CAD build for the part. Positions are in the model's coordinates, mm. Face numbers are marked on the shaded views. A direction names the side the tool comes from. Coordinates: 2 decimals unless noted, no trailing zeros. Loops run counter-clockwise (first coordinate to the right, second up) from the corner with the lowest first, then second, coordinate; pieces in that order, holes last. Notation, with made-up numbers: (-29.75, 51) -> (-25.75, 51) arc R31 cw to (-25.75, 86) -> close; hole circle Ø10 at (84, 88). An arc over 180 degrees is marked (long way). Write each question's results on one line, items separated by ' | '.
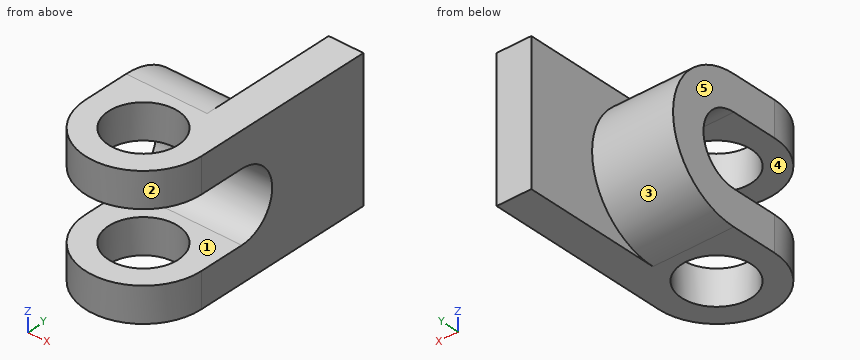
```python
from build123d import *

# Parameters (mm, degrees)
SKETCH1_R           = 15
BOSS_EXTRUDE1_DEPTH = 60
BOSS_EXTRUDE2_DEPTH = 35
CUT_EXTRUDE9_DEPTH  = 68


with BuildPart() as part:
    # Sketch1 → Boss-Extrude1 (new body)
    with BuildSketch(Plane.XY):
        with BuildLine():
            Line((25, 0), (25, 80))
            Line((25, 80), (10, 80))
            Line((10, 80), (10, 20))
            Line((10, 20), (-25, 20))
            Line((-25, 20), (-25, 0))
            ThreePointArc((-25, 0), (0, -25), (25, 0))
        make_face()
        Circle(SKETCH1_R, mode=Mode.SUBTRACT)
    extrude(amount=BOSS_EXTRUDE1_DEPTH)

    # Sketch2 → Boss-Extrude2 (add)
    with BuildSketch(Plane.ZY.offset(25)):
        with BuildLine():
            Line((15, 20), (0, 20))
            ThreePointArc((0, 20), (30, 50), (60, 20))
            Line((60, 20), (45, 20))
            ThreePointArc((45, 20), (30, 35), (15, 20))
        make_face()
    extrude(amount=-BOSS_EXTRUDE2_DEPTH)

    # Sketch4 → Cut-Extrude9 (cut)
    with BuildSketch(Plane.ZY.offset(25)):
        with BuildLine():
            Line((15, 20), (15, -31.386315339))
            Line((15, -31.386315339), (45, -31.386315339))
            Line((45, -31.386315339), (45, 20))
            ThreePointArc((45, 20), (30, 35), (15, 20))
        make_face()
    extrude(amount=-CUT_EXTRUDE9_DEPTH, mode=Mode.SUBTRACT)


solid = part.part
```
Q1. Pull direction Z, two halves, no side cores. Call the marked faces 1, 2 and 3: +Z half, -Z half, draft (parallel to the pull), parting line (faces both ways), or undercut.
Results are:
face 1: undercut | face 2: draft | face 3: parting line
Q2. Cut at C-C on z = 9.5. Write the cut outline in (x, y), and give its area (3 significant figures).
Results are:
outline: (-25, 0) arc R25 ccw to (25, 0) -> (25, 80) -> (10, 80) -> (10, 41.9) -> (-25, 41.9) -> close; hole circle Ø30 at (0, 0) | area: 2,940 mm^2
Q3. Wall check: L1, parallel to Z at x = 10, y = -14; L2, parallel to X at y = 0, z = 55; L3, parallel to Y at x = 0, z = 52.5. Give the ranges that are in metal, low to high. Write a range as from..to.
Results are:
L1: 0..15, 45..60 | L2: -25..-15, 15..25 | L3: -25..-15, 15..39.84
Q4. Cut at A-A on x = 0. Write the cut outline in (y, z).
Results are:
outline: (-25, 0) -> (-15, 0) -> (-15, 15) -> (-25, 15) -> close; (-25, 45) -> (-15, 45) -> (-15, 60) -> (-25, 60) -> close; (15, 0) -> (20, 0) arc R30 ccw to (20, 60) -> (15, 60) -> (15, 45) -> (20, 45) arc R15 cw to (20, 15) -> (15, 15) -> close
Q5. Drop a flat-ended pin along its axis: pin 1 (12 mm diameter, centred on x = -18, z = 46.5, fed in from +Y). Give the stop position or say it passes through.
Results are:
pin 1: y = 48.1
Q6. Cut at B-B on y = -11. Write the cut outline in (x, z), and give its area (3 significant figures).
Results are:
outline: (-22.45, 0) -> (-10.2, 0) -> (-10.2, 15) -> (-22.45, 15) -> close; (-22.45, 45) -> (-10.2, 45) -> (-10.2, 60) -> (-22.45, 60) -> close; (10.2, 0) -> (22.45, 0) -> (22.45, 15) -> (10.2, 15) -> close; (10.2, 45) -> (22.45, 45) -> (22.45, 60) -> (10.2, 60) -> close | area: 735 mm^2
Q7. Which spindle directions (+Z, -Z, +X, -X, +Y, -Y) get a long thin tool onto all of the face, cutting with end or side? Do the marked faces 4 and 5. Say none if no direction does.
Results are:
face 4: +X, -X, -Y | face 5: +Z, -Z, -X, +Y, -Y
